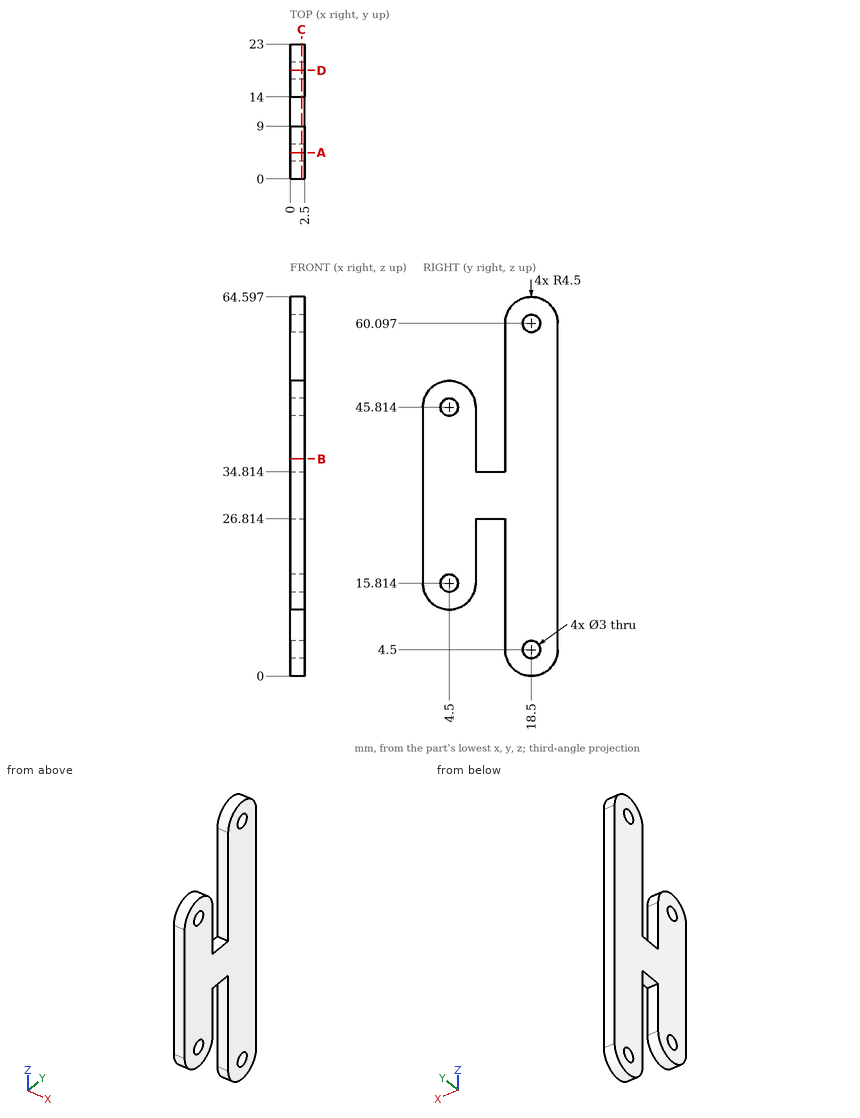
Job drawing, mm, ordinate dimensions from the low corner. One solid piece. Round coordinates to 2 decimals unless told otherwise and drop trailing zeros. Loops run counter-clockwise (first coordinate to the right, second up) from the corner with the lowest first, then second, coordinate; pieces in that order, holes last.
(1) Cut at D-D (y = 18.5). Give the cut face in (x, z).
(2) Drop flat-ended pins along their axis: pin 1 (1.2 mm diameter, centred on x = 1.5, y = 11.5, fed in from +Z); pin 2 (1.2 mm diameter, centred on x = 1.5, z = 47, fed in from -Y). Give the stop position or say it passes through.
(3) Cut at C-C (x = 1.95). Give the cut face in (y, z).
(4) Cut at A-A (y = 4.5). Give the cut face in (x, z).
(5) Cut at B-B (z = 37). Give the cut face in (x, y).
(6) Wall check: line 1 along Z through (x, y) = (1.75, 18.5); line 2 along Y through (x, z) = (2.05, 4.5); line 3 along Y through (x, z) = (1.9, 45.5). Give the ranges that are in metal, low to high.
Findings below:
1. outline: (0, 0) - (2.5, 0) - (2.5, 3) - (0, 3) - close; (0, 6) - (2.5, 6) - (2.5, 58.6) - (0, 58.6) - close; (0, 61.6) - (2.5, 61.6) - (2.5, 64.6) - (0, 64.6) - close
2. pin 1: stops at z = 34.81
2. pin 2: stops at y = 0.04
3. outline: (0, 15.81) arc R4.5 ccw to (9, 15.81) - (9, 26.81) - (14, 26.81) - (14, 4.5) arc R4.5 ccw to (23, 4.5) - (23, 60.1) arc R4.5 ccw to (14, 60.1) - (14, 34.81) - (9, 34.81) - (9, 45.81) arc R4.5 ccw to (0, 45.81) - close; hole circle Ø3 at (4.5, 15.81); hole circle Ø3 at (4.5, 45.81); hole circle Ø3 at (18.5, 4.5); hole circle Ø3 at (18.5, 60.1)
4. outline: (0, 11.31) - (2.5, 11.31) - (2.5, 14.31) - (0, 14.31) - close; (0, 17.31) - (2.5, 17.31) - (2.5, 44.31) - (0, 44.31) - close; (0, 47.31) - (2.5, 47.31) - (2.5, 50.31) - (0, 50.31) - close
5. outline: (0, 0) - (2.5, 0) - (2.5, 9) - (0, 9) - close; (0, 14) - (2.5, 14) - (2.5, 23) - (0, 23) - close
6. line 1: z = 0 to 3, 6 to 58.6, 61.6 to 64.6
6. line 2: y = 14 to 17, 20 to 23
6. line 3: y = 0 to 3.03, 5.97 to 9, 14 to 23
